Here's how the part is built. I have some questions about the finished solid (model axes, mm). Give positions to 0.01 mm unless a question says otherwise; leave off trailing zeros. Loops run counter-clockwise (first coordinate to the right, second up) from the corner with the lowest first, then second, coordinate; pieces in that order, holes last. Notation, with made-up numbers: (-20, -30.5) - (21, -30.5) arc R20 ccw to (21, 8.5) - close; hole circle Ø11 at (42, 6). An arc over 180 degrees is marked (long way). Return JSON: item names as keys, results as strings. Group by question number.
(1) For P1, Ø6, axis at y = 33.5, z = 85.5, coming from the -X side, with a flat end and sliding along its axis, tell me the tip position at first contact or that it passes through.
(2) If we section it at A-A (y = 38): Please give me the cut outline in (x, z), then the cut area to 3 significant figures.
(3) If we section it at C-C (x = 25): Please give me the cut outline in (y, z), then the cut area to 3 significant figures.
(4) If we section it at D-D (x = 6): Please give me the cut outline in (y, z).
(5) If we section it at B-B (z = 75): Please give me the cut outline in (x, y).
(6) I need wall thicknesses on probe 1 along X at (y, z) = (16.5, 25); probe 2 along Z at (x, y) = (31, 10); probe 3 along Y at (x, z) = (18.5, 75). Which ranges of each line are inside material? Lowest first, please. Write a range as [from, to].
(7) If we mould it in two halves opening along Z, with no side actions, what happens to faces 1 (the flat face through (25, 25, 100)), 2 (the flat face through (50, 25, 38)), 3 (the cylindrical face through (24.65, 25.83, 56.17)), 4 (the flat face through (25, 25, 0))? For each: released by +Z, released by -Z, zero draft, split by the parting line, or undercut.
```python
from build123d import *

# Parameters (mm, degrees)
SZKIC1_W                    = 50
SZKIC1_H                    = 50
DODANIE_WYCI_GNI_CIE1_DEPTH = 100
WYTNIJ_WYCI_GNI_CIE1_REACH  = 124.474
SZKIC2_R                    = 12.5
WYTNIJ_WYCI_GNI_CIE2_REACH  = 124.474
SZKIC3_R                    = 18.85


with BuildPart() as part:
    # Szkic1 → Dodanie-wyciągnięcie1 (new body)
    with BuildSketch(Plane.XY):
        with Locations((25, 25)):
            Rectangle(SZKIC1_W, SZKIC1_H)
    extrude(amount=DODANIE_WYCI_GNI_CIE1_DEPTH)

    # Szkic2 → Wytnij-wyciągnięcie1 (cut, up to next)
    with BuildSketch(Plane(origin=(0, 50, 0), x_dir=(1, 0, 0), z_dir=(0, 1, 0)), mode=Mode.PRIVATE) as wytnij_wyci_gni_cie1_sk1:
        with Locations(Location((25, -25, 0), (0, 0, 270))):
            Circle(SZKIC2_R)
    wytnij_wyci_gni_cie1_tool1 = extrude(wytnij_wyci_gni_cie1_sk1.sketch, amount=-WYTNIJ_WYCI_GNI_CIE1_REACH, mode=Mode.PRIVATE) & part.part
    add(wytnij_wyci_gni_cie1_tool1.solids().sort_by_distance((25, 50, 25))[0], mode=Mode.SUBTRACT)

    # Szkic3 → Wytnij-wyciągnięcie2 (cut, up to next)
    with BuildSketch(Plane.ZY, mode=Mode.PRIVATE) as wytnij_wyci_gni_cie2_sk1:
        with Locations((75, 25)):
            Circle(SZKIC3_R)
    wytnij_wyci_gni_cie2_tool1 = extrude(wytnij_wyci_gni_cie2_sk1.sketch, amount=-WYTNIJ_WYCI_GNI_CIE2_REACH, mode=Mode.PRIVATE) & part.part
    add(wytnij_wyci_gni_cie2_tool1.solids().sort_by_distance((0, 25, 75))[0], mode=Mode.SUBTRACT)


solid = part.part
```
Values:
{
 "1": {"P1": "through"},
 "2": {"outline": "(0, 0) - (50, 0) - (50, 61.35) - (0, 61.35) - close; (0, 88.65) - (50, 88.65) - (50, 100) - (0, 100) - close; hole circle Ø25 at (25, 25)", "area": "3,140 mm2"},
 "3": {"outline": "(0, 0) - (50, 0) - (50, 12.5) - (0, 12.5) - close; (0, 37.5) - (50, 37.5) - (50, 100) - (0, 100) - close; hole circle Ø37.7 at (25, 75)", "area": "2,630 mm2"},
 "4": {"outline": "(0, 0) - (50, 0) - (50, 100) - (0, 100) - close; hole circle Ø37.7 at (25, 75)"},
 "5": {"outline": "(0, 0) - (50, 0) - (50, 6.15) - (0, 6.15) - close; (0, 43.85) - (50, 43.85) - (50, 50) - (0, 50) - close"},
 "6": {"probe 1": "[0, 12.5], [37.5, 50]", "probe 2": "[0, 14.03], [35.97, 63.58], [86.42, 100]", "probe 3": "[0, 6.15], [43.85, 50]"},
 "7": {"face 1": "released by +Z", "face 2": "zero draft", "face 3": "undercut", "face 4": "released by -Z"}
}
